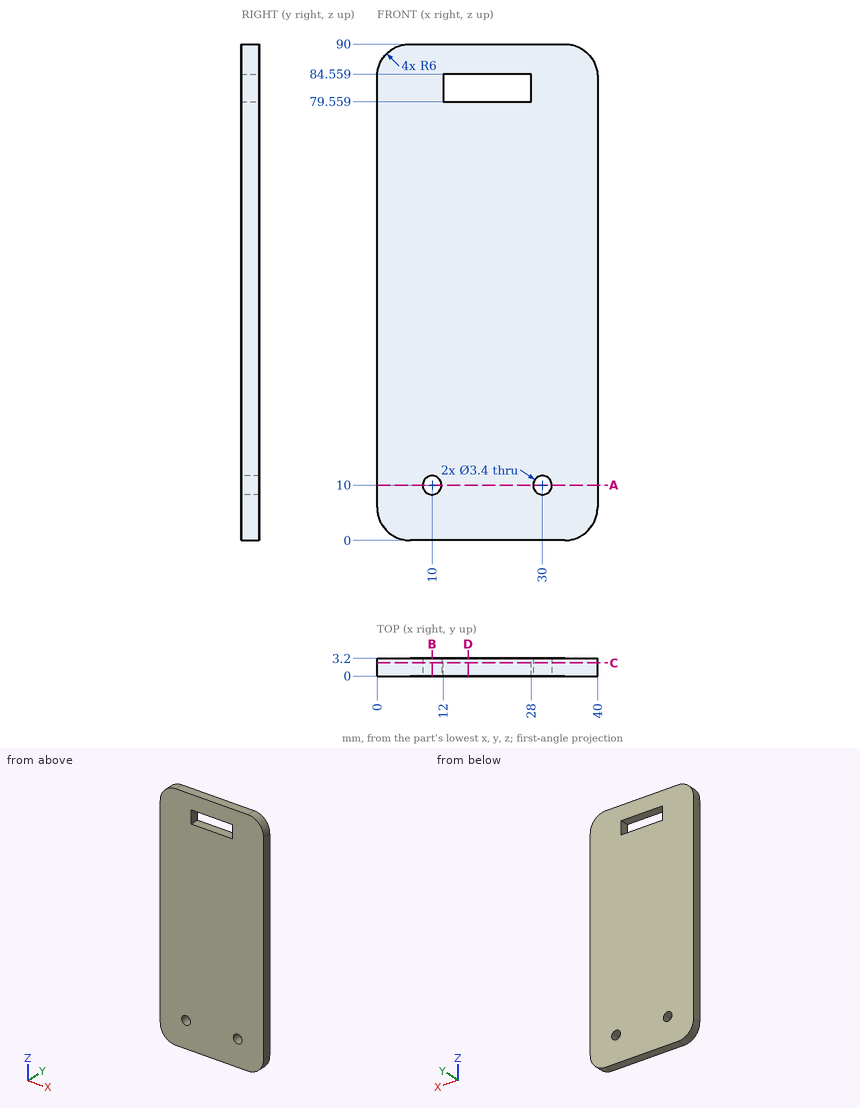
Print and shaded views of the part. All mm, measured from the part's lowest x, y and z. Give positions to 0.01 mm unless a question says otherwise; leave off trailing zeros. Loops run counter-clockwise (first coordinate to the right, second up) from the corner with the lowest first, then second, coordinate; pieces in that order, holes last. Notation, with made-up numbers: M 68,40.5 L 88,40.5 A30 ccw 88,68.5 Z; hole C -20,-1 d10. An arc over 180 degrees is marked long. Write each question's results on one line, items separated by ' | '.
Q1. Probe probe 1 along X at (y, z) = (1.35, 10); probe 2 along Z at (x, y) = (30, 1.45); probe 3 along Z at (x, y) = (13, 1.85). List the from-to ranges inside material, lowest first.
Geometry check:
probe 1: x = 0 to 8.3, 11.7 to 28.3, 31.7 to 40 | probe 2: z = 0 to 8.3, 11.7 to 90 | probe 3: z = 0 to 79.56, 84.56 to 90
Q2. Band-saw the part on B-B on x = 10. Write the cut outline in (y, z), and give its area (3 significant figures).
Geometry check:
outline: M 0,0 L 3.2,0 L 3.2,8.3 L 0,8.3 Z; M 0,11.7 L 3.2,11.7 L 3.2,90 L 0,90 Z | area: 277 mm²
Q3. Band-saw the part on C-C on y = 2.4. Write the cut outline in (x, z), and give its area (3 significant figures).
Geometry check:
outline: M 0,6 A6 ccw 6,0 L 34,0 A6 ccw 40,6 L 40,84 A6 ccw 34,90 L 6,90 A6 ccw 0,84 Z; hole C 10,10 d3.4; hole M 12,79.56 L 28,79.56 L 28,84.56 L 12,84.56 Z; hole C 30,10 d3.4 | area: 3,470 mm²
Q4. Band-saw the part on A-A on z = 10. Write the cut outline in (x, y), and give its area (3 significant figures).
Geometry check:
outline: M 0,0 L 8.3,0 L 8.3,3.2 L 0,3.2 Z; M 11.7,0 L 28.3,0 L 28.3,3.2 L 11.7,3.2 Z; M 31.7,0 L 40,0 L 40,3.2 L 31.7,3.2 Z | area: 106 mm²
Q5. Band-saw the part on D-D on x = 16.5. Write the cut outline in (y, z), and give its area (3 significant figures).
Geometry check:
outline: M 0,0 L 3.2,0 L 3.2,79.56 L 0,79.56 Z; M 0,84.56 L 3.2,84.56 L 3.2,90 L 0,90 Z | area: 272 mm²
